The figure shows three views and two pictorial views of one solid part (mm, origin at its lowest corner). Answer the questions. A direction names the side the tool comes from. Give positions to 0.01 mm unless a question says otherwise; leave off trailing zeros. Loops run counter-clockwise (first coordinate to the right, second up) from the corner with the lowest first, then second, coordinate; pieces in that order, holes last. Notation, with made-up numbers: (8.5, -25) -> (35.5, -25) arc R27 cw to (35.5, -4) -> close; hole circle Ø2 at (25, 77). An arc over 180 degrees is marked (long way). One line per item, written item: value. Start each with the question number.
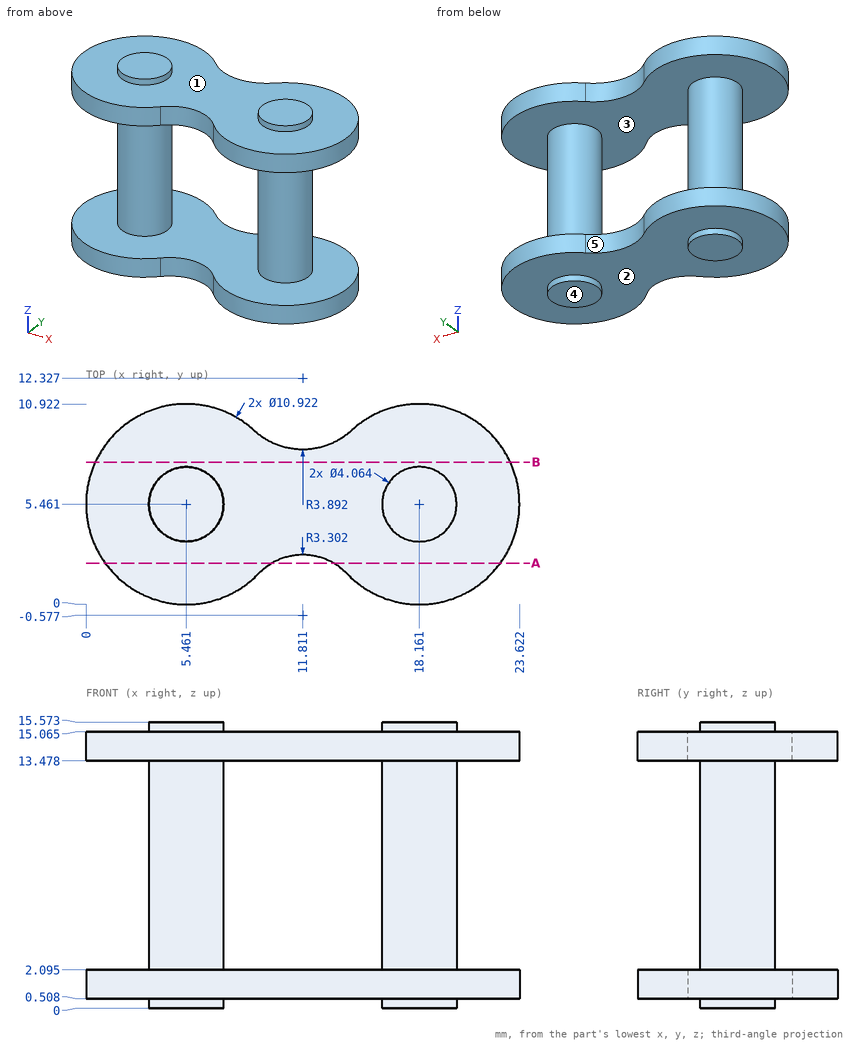
Item 1: For the marked faces 1, 2 and 3, determine the directions among +Z, -Z, +X, -X, +Y, -Y from which every point of the face is accessible in a straight line to the end or side of a thin tool.
Item 2: Section B-B, the plane y = 7.75 is taken. Determine the outline of the cut face in (x, z) (1 decimal).
Item 3: Consider L1, parallel to Z at x = 20.5, y = 1 (1 decimal); L2, parallel to X at y = 5.25, z = 4; L3, parallel to X at y = 7.25, z = 10.5 (1 decimal). Determine where each line is inside the solid, lowest interval first. Write a range as [from, to].
Item 4: Determine the mould class of the marked faces 4 and 5 for opening direction X: pulls with the +X half, pulls with the -X half, needs draft (parallel to the pull), parting line crosses it, or undercut.
Item 5: Section A-A, the plane y = 2.25 is taken. Determine the outline of the cut face in (x, z) (1 decimal).
Item 6: Flat-ended cylindrical pins translate along their axes: pin 1 (3.5 mm diameter, centred on x = 13.5, y = 4.5, fed in from +Z) (1 decimal); pin 2 (1 mm diameter, centred on y = 4.5, z = 2.5, fed in from +X); pin 3 (4 mm diameter, centred on x = 9.5, y = 2.5, fed in from -Z); pin 4 (8 mm diameter, centred on x = 18.5, z = 4.5, fed in from +Y). Find the tip coordinate at first contact, or state that the pin passes through.
Computed values:
1. face 1: +Z
1. face 2: -Z
1. face 3: none
2. outline: (0.5, 0.5) -> (23.1, 0.5) -> (23.1, 2.1) -> (0.5, 2.1) -> close; (0.5, 13.5) -> (23.1, 13.5) -> (23.1, 15.1) -> (0.5, 15.1) -> close
3. L1: [0.5, 2.1], [13.5, 15.1]
3. L2: [3.44, 7.48], [16.14, 20.18]
3. L3: [4.5, 6.4], [17.2, 19.1]
4. face 4: needs draft
4. face 5: undercut
5. outline: (1, 0.5) -> (10.1, 0.5) -> (10.1, 2.1) -> (1, 2.1) -> close; (1, 13.5) -> (10.1, 13.5) -> (10.1, 15.1) -> (1, 15.1) -> close; (13.5, 0.5) -> (22.6, 0.5) -> (22.6, 2.1) -> (13.5, 2.1) -> close; (13.5, 13.5) -> (22.6, 13.5) -> (22.6, 15.1) -> (13.5, 15.1) -> close
6. pin 1: z = 15.1
6. pin 2: x = 23.58
6. pin 3: z = 0.51
6. pin 4: y = 10.92
